from build123d import *

# Parameters (mm, degrees)
SKETCH1_W           = 25
SKETCH1_H           = 24
SKETCH1_R           = 1
BOSS_EXTRUDE1_DEPTH = 1
SKETCH2_W           = 8.5
SKETCH2_H           = 8.5
BOSS_EXTRUDE2_DEPTH = 2.5
SKETCH3_R           = 3.5
BOSS_EXTRUDE3_DEPTH = 2.2
SKETCH4_W           = 20
SKETCH4_H           = 6
BOSS_EXTRUDE4_DEPTH = 2.5


with BuildPart() as part:
    # Sketch1 → Boss-Extrude1 (new body)
    with BuildSketch(Plane(origin=(0, 0, 0), x_dir=(1, 0, 0), z_dir=(0, 1, 0))):
        with Locations((12.5, 12)):
            Rectangle(SKETCH1_W, SKETCH1_H)
        with Locations((2, 22)):
            Circle(SKETCH1_R, mode=Mode.SUBTRACT)
        with Locations((2, 9.5)):
            Circle(SKETCH1_R, mode=Mode.SUBTRACT)
        with Locations((23, 9.5)):
            Circle(SKETCH1_R, mode=Mode.SUBTRACT)
        with Locations((23, 22)):
            Circle(SKETCH1_R, mode=Mode.SUBTRACT)
    extrude(amount=BOSS_EXTRUDE1_DEPTH)

    # Sketch2 → Boss-Extrude2 (add)
    with BuildSketch(Plane(origin=(0, 1, 0), x_dir=(1, 0, 0), z_dir=(0, 1, 0))):
        with Locations((12.5, 12)):
            Rectangle(SKETCH2_W, SKETCH2_H)
    extrude(amount=BOSS_EXTRUDE2_DEPTH)

    # Sketch3 → Boss-Extrude3 (add)
    with BuildSketch(Plane(origin=(0, 3.5, 0), x_dir=(1, 0, 0), z_dir=(0, 1, 0))):
        with Locations((12.5, 12)):
            Circle(SKETCH3_R)
    extrude(amount=BOSS_EXTRUDE3_DEPTH)

    # Sketch4 → Boss-Extrude4 (add)
    with BuildSketch(Plane.XZ):
        with Locations((12.5, -3)):
            Rectangle(SKETCH4_W, SKETCH4_H)
    extrude(amount=BOSS_EXTRUDE4_DEPTH)


solid = part.part
Geometry check sheet. Reference: the model listing, model coordinates, mm. A direction names the side the tool comes from. Give positions to 0.01 mm unless a question says otherwise; leave off trailing zeros. Write each loop counter-clockwise with the first axis right and the second up, starting at its lowest first coordinate (ties: lowest second). Pieces come first, ordered by that corner, then holes. Notation, with made-up numbers: M -7,-24.5 L 5,-24.5 A27 cw 5,9.5 Z; hole C 13,-10.5 d11. An arc over 180 degrees is marked long. Answer as CSV lines item,"result". Start each with the question number.
Q1. Section check C-C, the plane z = -4. Record the cut outline in (x, y).
Q2. Material ranges on L1, parallel to Z at x = 2, y = 0.4; L2, parallel to X at y = 0.45, z = -22; L3, parallel to Y at x = 15, z = -18.5, recorded low to high.
Q3. Section check D-D, the plane x = 10.5. Record the cut outline in (y, z).
Q4. Go/stop test with flat-tipped pins: pin 1 (1.2 mm diameter, centred on y = -1, z = -3.5, fed in from +X); pin 2 (10 mm diameter, centred on x = 3, z = -17.5, fed in from -Y); pin 3 (1.2 mm diameter, centred on x = 14.5, y = 3, fed in from -Z). Record where each tip stops, or that it passes through.
Q5. Release check for a two-part mould opening along Z. For faces 1 (the face through (12, 0, -15)), 2 (the face through (1.783, 0.493, -21.024)), 3 (the face through (12, -1, -6)) record: pulls with the +Z half, pulls with the -Z half, needs draft (parallel to the pull), parting line crosses it, or undercut.
Q6. Tool access check on faces 4 (the face through (16.75, 2, -12)), 5 (the face through (22.5, -1, -3)), 6 (the face through (8.25, 2, -12)), 7 (the face through (12, 2, -7.75)). Record the directions out of +Z, -Z, +X, -X, +Y, -Y that give a thin tool (end or side, any length) a straight path to the whole face; none if there is none.
Q7. Section check A-A, the plane x = 2. Record the cut outline in (y, z), then the cut area to 3 significant figures.
Q8. Section check B-B, the plane z = -22. Record the cut outline in (x, y), then the cut area to 3 significant figures.
Geometry says:
1,outline,"M 0,0 L 2.5,0 L 2.5,-2.5 L 22.5,-2.5 L 22.5,0 L 25,0 L 25,1 L 0,1 Z"
2,L1,"-24 to -23, -21 to -10.5, -8.5 to 0"
2,L2,"0 to 1, 3 to 22, 24 to 25"
2,L3,"0 to 1"
3,outline,"M -2.5,-6 L 0,-6 L 0,-24 L 1,-24 L 1,-16.25 L 3.5,-16.25 L 3.5,-14.87 L 5.7,-14.87 L 5.7,-9.13 L 3.5,-9.13 L 3.5,-7.75 L 1,-7.75 L 1,0 L -2.5,0 Z"
4,pin 1,"x = 22.5"
4,pin 2,"y = 0"
4,pin 3,"z = -16.25"
5,face 1,"needs draft"
5,face 2,"undercut"
5,face 3,"pulls with the -Z half"
6,face 4,"+Z, -Z, +X, +Y"
6,face 5,"+Z, -Z, +X, -Y"
6,face 6,"+Z, -Z, -X, +Y"
6,face 7,"+Z, +X, -X, +Y"
7,outline,"M 0,-24 L 1,-24 L 1,-23 L 0,-23 Z; M 0,-21 L 1,-21 L 1,-10.5 L 0,-10.5 Z; M 0,-8.5 L 1,-8.5 L 1,0 L 0,0 Z"
7,area,"20.0 mm^2"
8,outline,"M 0,0 L 1,0 L 1,1 L 0,1 Z; M 3,0 L 22,0 L 22,1 L 3,1 Z; M 24,0 L 25,0 L 25,1 L 24,1 Z"
8,area,"21.0 mm^2"
